from build123d import *

# Parameters (mm, degrees)
PAD073_DEPTH       = 2
PAD074_DEPTH       = 3.5
SKETCH122_R        = 3.5
POCKET003054_DEPTH = 2.25
SKETCH123_R        = 4.702209
PAD075_DEPTH       = 2.2
SKETCH124_R        = 1.7
POCKET003055_DEPTH = 5
PAD076_DEPTH       = 3.5
SKETCH126_R        = 1.7
POCKET003056_DEPTH = 5
POCKET003057_DEPTH = 3
PAD078_DEPTH       = 4


with BuildPart() as obj1:
    # Sketch120 → Pad073 (new body, symmetric)
    with BuildSketch(Plane.XZ):
        with BuildLine():
            Line((7.19326, 28.01235), (20.118014, 28.01235))
            ThreePointArc((27.996703, 20.985646), (25.396468, 26.000474), (20.118014, 28.01235))
            Line((27.996703, 20.985646), (30.977077, -4.999855))
            Line((33.977077, -4.999855), (30.977077, -4.999855))
            Line((31.375084, 21.001564), (33.977077, -4.999855))
            ThreePointArc((31.375084, 21.001564), (27.724482, 28.375326), (20.118014, 31.51235))
            Line((7.19326, 31.51235), (20.118014, 31.51235))
            Line((7.19326, 28.01235), (7.19326, 31.51235))
        make_face()
    extrude(amount=PAD073_DEPTH, both=True)

    # Sketch121 → Pad074 (new body)
    with BuildSketch(Plane(origin=(0, 0, 31.51235), x_dir=(-1, 0, 0), z_dir=(0, 0, 1))):
        with BuildLine():
            Line((-18, 2), (-18, -2))
            Line((-18, -2), (-4.3876, -2))
            ThreePointArc((-4.3876, -2), (1.938593, -8.415251), (1.496731, 0.583689))
            ThreePointArc((1.496731, 0.583689), (-2.758605, 1.674941), (-7.139591, 2))
            Line((-18, 2), (-7.139591, 2))
        make_face()
    extrude(amount=-PAD074_DEPTH)

    # Sketch122 → Pocket003054 (cut)
    with BuildSketch(Plane(origin=(0, 0, 31.51235), x_dir=(-1, 0, 0), z_dir=(0, 0, 1))):
        with Locations((0, -4)):
            Circle(SKETCH122_R)
    extrude(amount=-POCKET003054_DEPTH, mode=Mode.SUBTRACT)

    # Sketch123 → Pad075 (new body)
    with BuildSketch(Plane(origin=(0, 0, 28.01235), x_dir=(1, 0, 0), z_dir=(0, 0, -1))):
        with Locations((-0.089106, -3.841625)):
            Circle(SKETCH123_R)
    extrude(amount=PAD075_DEPTH)

    # Sketch124 → Pocket003055 (cut)
    with BuildSketch(Plane(origin=(0, 0, 29.26235), x_dir=(-1, 0, 0), z_dir=(0, 0, 1))):
        with Locations((-0.080471, -3.899184)):
            Circle(SKETCH124_R)
    extrude(amount=-POCKET003055_DEPTH, mode=Mode.SUBTRACT)

    # Sketch125 → Pad076 (new body)
    with BuildSketch(Plane(origin=(0, 0, 31.51235), x_dir=(-1, 0, 0), z_dir=(0, 0, 1))):
        with BuildLine():
            Line((-22.021201, -1.987049), (-22.021201, -4.986919))
            ThreePointArc((-22.021201, -4.986919), (-17.510002, -9.511218), (-12.998803, -4.986919))
            Line((-12.998803, -4.986919), (-12.998803, -1.987049))
            Line((-22.021201, -1.987049), (-12.998803, -1.987049))
        make_face()
    extrude(amount=-PAD076_DEPTH)

    # Sketch126 → Pocket003056 (cut)
    with BuildSketch(Plane(origin=(0, 0, 31.51235), x_dir=(-1, 0, 0), z_dir=(0, 0, 1))):
        with Locations((-17.491917, -5)):
            Circle(SKETCH126_R)
    extrude(amount=-POCKET003056_DEPTH, mode=Mode.SUBTRACT)

    # Sketch127 → Pocket003057 (cut)
    with BuildSketch(Plane(origin=(0, 0, 31.51235), x_dir=(-1, 0, 0), z_dir=(0, 0, 1))):
        Polygon((-14.138998, -5.003928), (-15.835596, -2.057479), (-19.235593, -2.053552), (-20.938994, -4.996072), (-19.242396, -7.942521), (-15.842399, -7.946448), align=None)
    extrude(amount=-POCKET003057_DEPTH, mode=Mode.SUBTRACT)

    # Sketch128 → Pad078 (new body)
    with BuildSketch(Plane.XZ.offset(2)):
        with BuildLine():
            Line((27, 28.536497), (32.513573, -5))
            Line((32.513573, -5), (37.000002, -5))
            Line((37.000002, -5), (37.000002, -4.583553))
            ThreePointArc((33.505627, -1), (35.019116, -3.019659), (37.000002, -4.583553))
            Line((33, 5), (33.505627, -1))
            Line((35, 3.304739), (33, 5))
            Line((32.728943, 7), (35, 3.304739))
            Line((32, 13), (32.728943, 7))
            Line((34.496559, 10.608005), (32, 13))
            Line((32, 15), (34.496559, 10.608005))
            Line((31, 20), (32, 15))
            Line((33.606815, 17.606869), (31, 20))
            Line((31, 22), (33.606815, 17.606869))
            Line((27, 28.536497), (31, 22))
        make_face()
    extrude(amount=-PAD078_DEPTH)


with BuildPart() as part_mirroring013:
    # Part__Mirroring013: instance of obj1
    add(obj1.part.mirror(Plane(origin=(0, 0, 0), x_dir=(0, -1, 0), z_dir=(1, 0, 0))))


solid = part_mirroring013.part
Design review of the part built by this model. Coordinates are the model's own, in mm. A direction names the side the tool comes from. Give positions to 0.01 mm unless a question says otherwise; leave off trailing zeros. Write each loop counter-clockwise with the first axis right and the second up, starting at its lowest first coordinate (ties: lowest second). Pieces come first, ordered by that corner, then holes. Notation, with made-up numbers: M 86.25,78 L 91.25,78 A24 ccw 91.25,96 Z; hole C 55.25,-17 d4. An arc over 180 degrees is marked long. Return JSON: item names as keys, results as strings. Group by question number.
Item 1: Tool access review of faces 1 (the cylindrical face through (-25.457, -0.028, 25.946)), 2 (the cylindrical face through (-4.255, 5.643, 26.928)), 3 (the flat face through (-15.003, 6.496, 30.033)): name each direction out of +Z, -Z, +X, -X, +Y, -Y from which nothing blocks a thin tool from reaching the whole face with its end or side.
Item 2: Take a section at C-C (x = 0). Give the boundary of the cut face in (y, z), plus the area to 3 significant figures.
Item 3: Wall thickness on line 1 along X through (y, z) = (4, 31); line 2 along Z through (x, y) = (-20, 5); line 3 along X through (y, z) = (5, 28.2): over which ranges is each line inside the solid? List them lowest first.
Item 4: The part is to be moulded in two halves that separate along X. For faces 4 (the flat face through (-33.062, -0.028, 4.263)), 5 (the flat face through (-29.466, -0.028, 8.175)), 6 (the flat face through (-22.021, 3, 30)), say which applies: pulls with the +X half, pulls with the -X half, needs draft (parallel to the pull), parting line crosses it, or undercut.
Item 5: Clearance check with flat-ended pins moving along their axes: pin 1 Ø6.5 at (x, y) = (0, 4) entering from +Z; pin 2 Ø5 at (x, z) = (-28.5, 8.5) entering from +Y; pin 3 Ø3 at (x, y) = (-18, 3) entering from -Z. State where each tip first meets the part, or that it passes through.
Item 6: Take a section at D-D (z = 8). Give the boundary of the cut face in (x, y).
Item 7: Take a section at A-A (x = -16.5). Give the boundary of the cut face in (y, z).
Return value:
{
 "1": {"face 1": "-Z, +Y, -Y", "face 2": "-Z", "face 3": "+Z"},
 "2": {"outline": "M -1.06,28.01 L -0.86,28.01 L -0.86,25.81 L 2.2,25.81 L 2.2,29.26 L 0.5,29.26 L 0.5,31.51 L -1.06,31.51 Z; M 5.6,25.81 L 8.54,25.81 L 8.54,28.01 L 8.82,28.01 L 8.82,31.51 L 7.5,31.51 L 7.5,29.26 L 5.6,29.26 Z", "area": "27.8 mm2"},
 "3": {"line 1": "x = -22.02 to -20.36, -14.72 to -13, -4.82 to -3.5, 3.5 to 4.82", "line 2": "z = 28.01 to 28.51", "line 3": "x = -22.02 to -19.19, -15.79 to -13, -4.72 to -1.38, 1.21 to 4.72"},
 "4": {"face 4": "undercut", "face 5": "pulls with the +X half", "face 6": "pulls with the -X half"},
 "5": {"pin 1": "stops at z = 29.26", "pin 2": "stops at y = 2", "pin 3": "stops at z = 28.01"},
 "6": {"outline": "M -32.68,-2 L -29.49,-2 L -29.49,2 L -32.68,2 Z"},
 "7": {"outline": "M -2,28.01 L 3.62,28.01 L 3.62,28.51 L 2.06,28.51 L 2.06,31.51 L -2,31.51 Z; M 6.38,28.01 L 9.4,28.01 L 9.4,31.51 L 7.95,31.51 L 7.95,28.51 L 6.38,28.51 Z"}
}
